```python
from build123d import *

# Parameters (mm, degrees)
SKETCH_1_W              = 80
SKETCH_1_H              = 34
EXTRUDE_1_DEPTH         = 3
SKETCH_2_W              = 70
SKETCH_2_H              = 23
CUT_EXTRUDE_2_DEPTH     = 3
CHAMFER_1_SIZE          = 0.5
SKETCH_7_W              = 25
SKETCH_7_H              = 3
CUT_EXTRUDE_6_DEPTH     = 3
FILLET_2_R              = 2
CHAMFER_2_SIZE          = 11
CHAMFER_2_SIZE2         = 6.350852961
CHAMFER_3_SIZE          = 11
CHAMFER_3_SIZE2         = 6.350852961
FILLET_3_R              = 2
HOLE_WIZARD_2_5_2_5_1_D = 2.5
SKETCH_11_W             = 69
SKETCH_11_H             = 10.181057749
CUT_EXTRUDE_1_DEPTH     = 10
EXTRUDE_2_DEPTH         = 3
EXTRUDE_4_DEPTH         = 3
EXTRUDE_5_DEPTH         = 31


with BuildPart() as part:
    # 草图1 → Extrude 1 (new body)
    with BuildSketch(Plane.XY):
        Rectangle(SKETCH_1_W, SKETCH_1_H)
    extrude(amount=EXTRUDE_1_DEPTH)

    # 草图2 → 拉伸2 (cut)
    with BuildSketch(Plane.XY.offset(3)):
        Rectangle(SKETCH_2_W, SKETCH_2_H)
    extrude(amount=-CUT_EXTRUDE_2_DEPTH, mode=Mode.SUBTRACT)

    # 倒角1
    chamfer_1_edges = [part.edges().sort_by_distance(p)[0] for p in [
        (-40, 17, 1.5),
        (40, 17, 1.5),
    ]]
    chamfer(chamfer_1_edges, length=CHAMFER_1_SIZE)

    # 草图7 → 拉伸6 (cut)
    with BuildSketch(Plane.XY.offset(3)):
        with Locations((0, -15.5)):
            Rectangle(SKETCH_7_W, SKETCH_7_H)
    extrude(amount=-CUT_EXTRUDE_6_DEPTH, mode=Mode.SUBTRACT)

    # 圆角2
    fillet_2_edges = [part.edges().sort_by_distance(p)[0] for p in [
        (-12.5, -14, 1.5),
        (12.5, -14, 1.5),
    ]]
    fillet(fillet_2_edges, radius=FILLET_2_R)

    # 倒角2
    chamfer_2_edges = [part.edges().sort_by_distance(p)[0] for p in [
        (40, -17, 1.5),
    ]]
    chamfer_2_side = [part.faces().sort_by_distance(p)[0] for p in [
        (26.25, -17, 1.5),
    ]]
    chamfer(chamfer_2_edges, length=CHAMFER_2_SIZE, length2=CHAMFER_2_SIZE2, reference=chamfer_2_side[0])

    # 倒角3
    chamfer_3_edges = [part.edges().sort_by_distance(p)[0] for p in [
        (-40, -17, 1.5),
    ]]
    chamfer_3_side = [part.faces().sort_by_distance(p)[0] for p in [
        (-26.25, -17, 1.5),
    ]]
    chamfer(chamfer_3_edges, length=CHAMFER_3_SIZE, length2=CHAMFER_3_SIZE2, reference=chamfer_3_side[0])

    # 圆角3
    fillet_3_edges = [part.edges().sort_by_distance(p)[0] for p in [
        (12.5, -17, 1.5),
        (-12.5, -17, 1.5),
    ]]
    fillet(fillet_3_edges, radius=FILLET_3_R)

    # Ø2.5 (2.5) 直径孔1 (through all)
    with Locations(Plane(origin=(-37.5, -7, 0), x_dir=(-1, 0, 0), z_dir=(0, 0, -1))):
        with Locations((0, 0), (0, 21), (-75, 21), (-75, 0)):
            Hole(HOLE_WIZARD_2_5_2_5_1_D / 2)

    # 草图11 → 切除-拉伸1 (cut)
    with BuildSketch(Plane.XY.offset(3)):
        with Locations((0, -18.915102393)):
            Rectangle(SKETCH_11_W, SKETCH_11_H)
    extrude(amount=-CUT_EXTRUDE_1_DEPTH, mode=Mode.SUBTRACT)

    # 草图12 → 凸台-拉伸2 (add)
    with BuildSketch(Plane.XY.offset(3)):
        Polygon((-40, -10.649147039), (-34.5, -13.824573519), (34.5, -13.824573519), (40, -10.649147039), (35, -14.3), (-35, -14.3), align=None)
    extrude(amount=-EXTRUDE_2_DEPTH)

    # 草图13 → 凸台-拉伸4 (add)
    with BuildSketch(Plane.XY.offset(3)):
        Polygon((-35, -11.5), (-35, -9.5), (35, -9.5), (35, -11.9), (-35, -11.9), align=None)
    extrude(amount=-EXTRUDE_4_DEPTH)

    # 草图13<2> → 凸台-拉伸5 (add)
    with BuildSketch(Plane.XY.offset(3)):
        Polygon((-35, -11.5), (-35, -9.5), (35, -9.5), (35, -11.9), (-35, -11.9), align=None)
    extrude(amount=EXTRUDE_5_DEPTH)


solid = part.part
```
Geometry: final body of the model. Coordinates: model frame, mm. A direction names the side the tool comes from. Coordinates: 2 decimals unless noted, no trailing zeros. Write each loop counter-clockwise with the first axis right and the second up, starting at its lowest first coordinate (ties: lowest second). Pieces come first, ordered by that corner, then holes. Notation, with made-up numbers: M 61,-13 L 86,-13 A19 cw 86,20 Z; hole C 51,34 d6. An arc over 180 degrees is marked long. Answer as CSV lines item,"result". Start each with the question number.
Q1. Cut plane A-A on y = 7.5. Return the cut outline in (x, z), then the cut area to 3 significant figures.
Q2. Cut plane D-D on y = -7. Return the cut outline in (x, z).
Q3. Line query: line 1 (Y direction, x = 37.5, z = 2); line 2 (Y direction, x = -28, z = 20). Output: solid intervals per line, ascending. Write a range as from..to.
Q4. Mould query, pull axis Y, two halves, no side actions, for faces 1 (the flat face through (-1, 17, 1)), 2 (the flat face through (37.535, -12.449, 1.521)), 3 (the cylindrical face through (36.579, 14.845, 1.521)). Classes: released by +Y, released by -Y, zero draft, split by the parting line, or undercut.
Q5. Cut plane B-B on y = 14. Return the cut outline in (x, z), then the cut area to 3 significant figures.
Q6. Reachability of faces 4 (the flat face through (-35, 1, 2)), 5 (the flat face through (-35, -11, 18)), 6 (the flat face through (0, -11.9, 18)) from +Z, -Z, +X, -X, +Y, -Y: full face, straight path, thin tool, end or side. Return the list, or none.
Q7. Pin query (flat end, axial travel): P1, Ø12, axis at x = -14, y = 13, coming from the +Z side; P2, Ø12, axis at x = -3, z = 18.5, coming from the -Y side; P3, Ø6, axis at y = -9.5, z = 10.5, coming from the -X side. Return the tip coordinate at first contact, or that it passes through.
Q8. Cut plane C-C on x = 21.5. Return the cut outline in (y, z).
Findings below:
1,outline,"M -40,0 L -35,0 L -35,3 L -40,3 Z; M 35,0 L 40,0 L 40,3 L 35,3 Z"
1,area,"30.0 mm2"
2,outline,"M -40,0 L -38.75,0 L -38.75,3 L -40,3 Z; M -36.25,0 L -35,0 L -35,3 L -36.25,3 Z; M 35,0 L 36.25,0 L 36.25,3 L 35,3 Z; M 38.75,0 L 40,0 L 40,3 L 38.75,3 Z"
3,line 1,"y = -12.47..-8.25, -5.75..12.75, 15.25..17"
3,line 2,"y = -11.9..-9.5"
4,face 1,"released by +Y"
4,face 2,"released by -Y"
4,face 3,"undercut"
5,outline,"M -40,0 L -38.75,0 L -38.75,3 L -40,3 Z; M -36.25,0 L 36.25,0 L 36.25,3 L -36.25,3 Z; M 38.75,0 L 40,0 L 40,3 L 38.75,3 Z"
5,area,"225 mm2"
6,face 4,"+Z, -Z"
6,face 5,"+Z, -X, +Y, -Y"
6,face 6,"+Z, +X, -X, -Y"
7,P1,"stops at z = 3"
7,P2,"stops at y = -11.9"
7,P3,"stops at x = -35"
8,outline,"M -14.3,0 L -9.5,0 L -9.5,34 L -11.9,34 L -11.9,3 L -14.3,3 Z; M 11.5,0 L 17,0 L 17,3 L 11.5,3 Z"
